from build123d import *

# Parameters (mm, degrees)
SKETCH_1_R          = 1.7
EXTRUDE_1_DEPTH     = 39
FILLET_1_R          = 10
EXTRUDE_2_DEPTH     = 5
EXTRUDE_START       = -3
SKETCH_4_R          = 1.7
EXTRUDE_3_DEPTH     = 3
CUT_EXTRUDE_2_DEPTH = 5
SKETCH_6_R          = 1.7
EXTRUDE_4_DEPTH     = 3
SKETCH_7_R          = 1.7
EXTRUDE_5_DEPTH     = 5
SKETCH_8_R          = 3
SKETCH_8_R_2        = 1.7
EXTRUDE_6_DEPTH     = 39


with BuildPart() as part:
    # 草图1 → 凸台-拉伸1 (new body)
    with BuildSketch(Plane(origin=(0, 0, 0), x_dir=(1, 0, 0), z_dir=(0, 1, 0))):
        with BuildLine():
            Line((-14.277701198, -3), (35.505461262, -3))
            ThreePointArc((35.505461262, -3), (36.773316047, -2.718923361), (37.803594591, -1.928362829))
            Line((37.803594591, -1.928362829), (63.497014217, 28.691862316))
            Line((63.497014217, 28.691862316), (61.198880888, 30.620225145))
            Line((61.198880888, 30.620225145), (37.433824091, 2.298133329))
            ThreePointArc((37.433824091, 2.298133329), (34.237606477, 2.718923361), (32.505461262, 0))
            Line((32.505461262, 0), (-11.277701198, 0))
            ThreePointArc((-11.277701198, 0), (-16.399021541, 2.121320344), (-14.277701198, -3))
        make_face()
        with Locations(Location((-14.277701198, 0, 0), (0, 0, 270))):
            Circle(SKETCH_1_R, mode=Mode.SUBTRACT)
        with Locations(Location((35.505461262, 0, 0), (0, 0, 270))):
            Circle(SKETCH_1_R, mode=Mode.SUBTRACT)
    extrude(amount=EXTRUDE_1_DEPTH)

    # 圆角1
    fillet_1_edges = [part.edges().sort_by_distance(p)[0] for p in [
        (37.433824091, 19.5, -2.298133329),
        (-11.277701198, 19.5, 0),
        (32.505461262, 19.5, 0),
    ]]
    fillet(fillet_1_edges, radius=FILLET_1_R)

    # 草图3 → 凸台-拉伸2 (add)
    with BuildSketch(Plane(origin=(0, 0, 0), x_dir=(1, 0, 0), z_dir=(0, 1, 0))):
        with BuildLine():
            Line((-14.277701198, 3), (35.505461262, 3))
            ThreePointArc((35.505461262, 3), (38.505461262, 0), (35.505461262, -3))
            Line((35.505461262, -3), (-14.277701198, -3))
            ThreePointArc((-14.277701198, -3), (-17.277701198, 0), (-14.277701198, 3))
        make_face()
    extrude(amount=EXTRUDE_2_DEPTH)

    # 草图4 → 凸台-拉伸3 (add)
    with BuildSketch(Plane(origin=(0, 39, 0), x_dir=(1, 0, 0), z_dir=(0, 1, 0)).offset(EXTRUDE_START)):
        with BuildLine():
            Line((-14.277701198, 3), (35.505461262, 3))
            ThreePointArc((35.505461262, 3), (38.505461262, 0), (35.505461262, -3))
            Line((35.505461262, -3), (-14.277701198, -3))
            ThreePointArc((-14.277701198, -3), (-17.277701198, 0), (-14.277701198, 3))
        make_face()
        with Locations(Location((-14.277701198, 0, 0), (0, 0, 270))):
            Circle(SKETCH_4_R, mode=Mode.SUBTRACT)
        with Locations(Location((35.505461262, 0, 0), (0, 0, 270))):
            Circle(SKETCH_4_R, mode=Mode.SUBTRACT)
    extrude(amount=EXTRUDE_3_DEPTH)

    # 草图5 → 切除-拉伸2 (cut)
    with BuildSketch(Plane.XY.offset(3)):
        with BuildLine():
            Line((-2.386119968, 30.5), (23.613880032, 30.5))
            ThreePointArc((23.613880032, 30.5), (26.613880032, 27.5), (23.613880032, 24.5))
            Line((23.613880032, 24.5), (-2.386119968, 24.5))
            ThreePointArc((-2.386119968, 24.5), (-5.386119968, 27.5), (-2.386119968, 30.5))
        make_face()
        with BuildLine():
            Line((-2.386119968, 8.5), (23.613880032, 8.5))
            ThreePointArc((23.613880032, 8.5), (26.613880032, 11.5), (23.613880032, 14.5))
            Line((23.613880032, 14.5), (-2.386119968, 14.5))
            ThreePointArc((-2.386119968, 14.5), (-5.386119968, 11.5), (-2.386119968, 8.5))
        make_face()
    extrude(amount=-CUT_EXTRUDE_2_DEPTH, mode=Mode.SUBTRACT)

    # 草图6 → 凸台-拉伸4 (add)
    with BuildSketch(Plane(origin=(0, 39, 0), x_dir=(1, 0, 0), z_dir=(0, 1, 0)).offset(EXTRUDE_START)):
        with BuildLine():
            Line((33.207327933, 1.928362829), (58.890388489, 32.536242516))
            ThreePointArc((58.890388489, 32.536242516), (63.116884647, 32.906013016), (63.486655148, 28.679516858))
            Line((63.486655148, 28.679516858), (37.803594591, -1.928362829))
            ThreePointArc((37.803594591, -1.928362829), (33.577098433, -2.298133329), (33.207327933, 1.928362829))
        make_face()
        with Locations(Location((35.505461262, 0, 0), (0, 0, 270))):
            Circle(SKETCH_6_R, mode=Mode.SUBTRACT)
        with Locations((61.188521818, 30.607879687)):
            Circle(SKETCH_6_R, mode=Mode.SUBTRACT)
    extrude(amount=EXTRUDE_4_DEPTH)

    # 草图7 → 凸台-拉伸5 (add)
    with BuildSketch(Plane(origin=(0, 0, 0), x_dir=(1, 0, 0), z_dir=(0, 1, 0))):
        with BuildLine():
            Line((33.207327933, 1.928362829), (58.890388489, 32.536242516))
            ThreePointArc((58.890388489, 32.536242516), (63.116884647, 32.906013016), (63.486655148, 28.679516858))
            Line((63.486655148, 28.679516858), (37.803594591, -1.928362829))
            ThreePointArc((37.803594591, -1.928362829), (33.577098433, -2.298133329), (33.207327933, 1.928362829))
        make_face()
        with Locations(Location((35.505461262, 0, 0), (0, 0, 270))):
            Circle(SKETCH_7_R, mode=Mode.SUBTRACT)
        with Locations((61.188521818, 30.607879687)):
            Circle(SKETCH_7_R, mode=Mode.SUBTRACT)
    extrude(amount=EXTRUDE_5_DEPTH)

    # 草图8 → 凸台-拉伸6 (add)
    with BuildSketch(Plane(origin=(0, 0, 0), x_dir=(1, 0, 0), z_dir=(0, 1, 0))):
        with Locations((61.188521818, 30.607879687)):
            Circle(SKETCH_8_R)
        with Locations((61.188521818, 30.607879687)):
            Circle(SKETCH_8_R_2, mode=Mode.SUBTRACT)
    extrude(amount=EXTRUDE_6_DEPTH)


solid = part.part
CAD build for the part. Positions are in the model's coordinates, mm. A direction names the side the tool comes from. Coordinates: 2 decimals unless noted, no trailing zeros. Order: outer loops, then holes, each group sorted by start corner. A loop starts at its lowest first (then second) coordinate and runs counter-clockwise, first axis right, second up.
Item 1: Band-saw the part on A-A on y = 27.5. Give the number of separate pieces and of enclosed holes in the cut face, plus the area to 3 significant figures.
Check sheet entries:
separate pieces: 2
enclosed holes: 3
area: 214 mm2
Item 2: Band-saw the part on B-B on x = 20. List the corners of the cut face in (y, z), plus the area to 3 significant figures.
Check sheet entries:
outline: (0, -3) - (5, -3) - (5, 0) - (8.5, 0) - (8.5, 3) - (0, 3) - close; (14.5, 0) - (24.5, 0) - (24.5, 3) - (14.5, 3) - close; (30.5, 0) - (36, 0) - (36, -3) - (39, -3) - (39, 3) - (30.5, 3) - close
area: 105 mm2
Item 3: 3-axis set-ups, long thin cutter, end or side, ignore diameter. For faces 1 (the face through (-17.071, 19.227, -1.094)), 2 (the face through (50.5, 19.2, -13.2)), 3 (the face through (11, 24, 0)), 4 (the face through (26.613, 27.566, 1.521)): which of +Z, -Z, +X, -X, +Y, -Y reach the whole face in a straight line?
Check sheet entries:
face 1: none
face 2: +Z, +X, +Y, -Y
face 3: -Z
face 4: +Z, -Z
Item 4: Drill centre lines: L1, parallel to Y at x = 2, z = -1.5; L2, parallel to Z at x = -12, y = 4.5; L3, parallel to Z at x = -13, y = 12.5. Where is each one in solid material? Low to high.
Check sheet entries:
L1: y = 0 to 5, 36 to 39
L2: z = -3 to 3
L3: z = -2.71 to -1.12, 1.12 to 3
Item 5: Pin check, flat tips, straight feed: pin 1 Ø1.5 at (y, z) = (17, -18) entering from +X; pin 2 Ø1 at (x, y) = (38.5, 12) entering from -Z; pin 3 Ø2.5 at (x, z) = (35.51, 0) entering from +Y. Stop position of each tip, or through.
Check sheet entries:
pin 1: stops at x = 55.15
pin 2: stops at z = -4.66
pin 3: stops at y = 5
Item 6: Two-plate mould, pull along Y, no slides. Class faces 5 (the face through (10, 37, -3)), 6 (the face through (27, 0, -2)), 7 (the face through (-9.41, 20.72, -0.61)), 8 (the face through (38.164, 20.717, -4.119)): +Y half, -Y half, draft (parallel to the pull), parting line (faces both ways), or undercut.
Check sheet entries:
face 5: draft
face 6: -Y half
face 7: undercut
face 8: undercut
